Input: part model. Units: mm. Frame: model coordinates. A direction names the side the tool comes from. Coordinates: 2 decimals unless noted, no trailing zeros. Write each loop counter-clockwise with the first axis right and the second up, starting at its lowest first coordinate (ties: lowest second). Pieces come first, ordered by that corner, then holes. Notation, with made-up numbers: (43, 4) - (84, 4) arc R11 cw to (84, 11) - close; hole circle Ø3 at (9.25, 39.5). An arc over 180 degrees is marked (long way). Put each result on its own line as item: value. Start each with the question number.
1. Pull-direction query (Y, two-part tool) for faces 1 (the flat face through (7.5, 0, 0)), 2 (the cylindrical face through (36.98, 11.26, -35.77)), 3 (the flat face through (75, 25, 17)); classes: released by +Y, released by -Y, zero draft, split by the parting line, or undercut.
2. Access query for faces 4 (the flat face through (0, 1, 1)), 5 (the cylindrical face through (40.777, -11.49, -27.712)). Directions: +Z, -Z, +X, -X, +Y, -Y. A direction counts if a zero-diameter tool reaches every point of the face in a straight line with its end or side. Return the directions, or none.
3. Cut plane D-D, the plane x = 17. Return loops of the section in (y, z).
4. Cut plane A-A, the plane y = 0. Return loops of the section in (x, z).
5. Cut plane C-C, the plane z = 0. Return loops of the section in (x, y).
6. Pin query (flat end, axial travel): pin 1 (1 mm diameter, centred on x = 50.5, z = 10, fed in from -Y); pin 2 (9 mm diameter, centred on x = 37.5, y = 0, fed in from +Z); pin 3 (6 mm diameter, centred on x = 9, y = -9.5, fed in from +Z); pin 4 (2 mm diameter, centred on x = 42.5, z = 19.5, fed in from +Y). Return the tip coordinate at first contact, or that it passes through.
7. Line query: line 1 (X direction, y = 0, z = -34.25); line 2 (Z direction, x = 21, y = 0). Output: solid intervals per line, ascending.
8. Cut plane B-B, the plane x = 33. Return loops of the section in (y, z).
from build123d import *

# Parameters (mm, degrees)
SKETCH1_R               = 37.5
BOSS_EXTRUDE1_DEPTH     = 75
SHELL1_T                = -7.5
SKETCH2_R               = 7.5
CUT_EXTRUDE1_DEPTH      = 92.855865354
CUT_EXTRUDE1_DEPTH_BACK = 92.855865354


with BuildPart() as part:
    # Sketch1 → Boss-Extrude1 (new body)
    with BuildSketch(Plane(origin=(0, 0, 0), x_dir=(0, 0, -1), z_dir=(1, 0, 0))):
        Circle(SKETCH1_R)
    extrude(amount=BOSS_EXTRUDE1_DEPTH)

    # Shell1
    shell1_openings = [part.faces().sort_by_distance(p)[0] for p in [
        (75, 0, 0),
    ]]
    offset(amount=SHELL1_T, openings=shell1_openings, kind=Kind.INTERSECTION)

    # Sketch2 → Cut-Extrude1 (cut, two sides)
    with BuildSketch(Plane.XY) as cut_extrude1_sk:
        with Locations((37.5, 0)):
            Circle(SKETCH2_R)
    extrude(amount=CUT_EXTRUDE1_DEPTH, mode=Mode.SUBTRACT)
    extrude(cut_extrude1_sk.sketch, amount=-CUT_EXTRUDE1_DEPTH_BACK, mode=Mode.SUBTRACT)


solid = part.part
Report:
1. face 1: undercut
1. face 2: split by the parting line
1. face 3: zero draft
2. face 4: +Z, -Z, -X, +Y, -Y
2. face 5: +X
3. outline: circle Ø75 at (0, 0); hole circle Ø60 at (0, 0)
4. outline: (0, -37.5) - (30, -37.5) - (30, -30) - (7.5, -30) - (7.5, 30) - (30, 30) - (30, 37.5) - (0, 37.5) - close; (45, -37.5) - (75, -37.5) - (75, -30) - (45, -30) - close; (45, 30) - (75, 30) - (75, 37.5) - (45, 37.5) - close
5. outline: (0, -37.5) - (75, -37.5) - (75, -30) - (7.5, -30) - (7.5, 30) - (75, 30) - (75, 37.5) - (0, 37.5) - close
6. pin 1: stops at y = -36.28
6. pin 2: passes through
6. pin 3: stops at z = 36.93
6. pin 4: stops at y = 32.62
7. line 1: x = 0 to 30, 45 to 75
7. line 2: z = -37.5 to -30, 30 to 37.5
8. outline: (-6, -37.02) - (-6, -29.39) arc R30 cw to (-6, 29.39) - (-6, 37.02) arc R37.5 ccw to start; (6, -37.02) arc R37.5 ccw to (6, 37.02) - (6, 29.39) arc R30 cw to (6, -29.39) - close
